Solid Edge part; units mm, degrees
sketch "Sketch1" plane through (0, 0, 0) normal (0, -1, 0) x (1, 0, 0)
  line L0 (-39.1421, 0) -> (39.1421, 0)
  line L1 (39.1421, 0) -> (91.1421, 52)
  line L2 (91.1421, 52) -> (77, 52)
  line L3 (77, 52) -> (30, 5)
  line L4 (30, 5) -> (-30, 5)
  line L5 (-30, 5) -> (-77, 52)
  line L6 (-77, 52) -> (-91.1421, 52)
  line L7 (-91.1421, 52) -> (-39.1421, 0)
  dimension "D1" = 30
extrude "Protrusion1" add sketch "Sketch1" along normal blind 94.9203
sketch "Sketch2" plane through (0, -94.9203, 21) normal (0, -1, 0) x (1, 0, 0)
  line L0 (-86.1421, 26) -> (-91.1421, 31)
  line L1 (-101.1421, 26) -> (-86.1421, 26)
  line L2 (-101.1421, 31) -> (-101.1421, 26)
  line L3 (-91.1421, 31) -> (-101.1421, 31)
  dimension "D1" = 91.1421
  dimension "D2" = 101.1421
extrude "Protrusion2" add sketch "Sketch2" against normal up to vertex (94.9203 mm away)
mirror "Mirror1" about plane through (0, 0, 0) normal (1, 0, 0) of "Protrusion2"
sketch "Sketch3" plane through (0, -47.4602, 5) normal (0, 0, 1) x (1, 0, 0)
  circle A0 centre (-16, 21) radius 2
  circle A1 centre (-16, -21) radius 2
  circle A2 centre (16, -21) radius 2
  circle A3 centre (16, 21) radius 2
  dimension "D1" = 16
  dimension "D2" = 16
extrude "Cutout1" cut sketch "Sketch3" against normal through all
sketch "Sketch4" plane through (-78.2221, -47.4602, 52) normal (0, 0, 1) x (1, 0, 0)
  circle A0 centre (-17.7801, -40) radius 1.5
  circle A1 centre (174.2242, -40) radius 1.5
  circle A2 centre (174.2242, 40) radius 1.5
  circle A3 centre (-17.7801, 40) radius 1.5
  dimension "D1" = 17.7801
extrude "Cutout2" cut sketch "Sketch4" against normal through all
properties material "Nylon, allgemein"
The model under review builds one solid part; all positions refer to its coordinate system, in mm. A direction names the side the tool comes from. Round coordinates to 2 decimals unless told otherwise and drop trailing zeros. Loops run counter-clockwise (first coordinate to the right, second up) from the corner with the lowest first, then second, coordinate; pieces in that order, holes last. Notation, with made-up numbers: (28, 59.5) -> (32, 59.5) arc R13 ccw to (32, 71.5) -> close; hole circle Ø9 at (-9.5, 10). An arc over 180 degrees is marked (long way). Answer as a JSON object with one key per item and string values. Group by question number.
1) For faces 1 (the face through (0, -47, 5)), 2 (the face through (-94, -48, 47)), 3 (the face through (-1, -47, 0)), 4 (the face through (94, -48, 47)), list the 3-axis set-ups (+Z, -Z, +X, -X, +Y, -Y) from which the entire face can be reached by the end or side of a thin tool; tool diameter is ignored.
2) We need section D-D on x = 34. Write out the cut boundary in (y, z), then the cut area to 3 significant figures.
3) For pin 1 Ø7.5 at (x, y) = (-93.5, -56.5) entering from -Z; pin 2 Ø5 at (y, z) = (-81.5, 33.5) entering from +X; pin 3 Ø4 at (y, z) = (-20.5, 28) entering from +X, all flat-tipped, find the tip position at first contact; note any pin that passes through.
4) We need section C-C on z = 43. Write out the cut boundary in (x, y), then the cut area to 3 significant figures.
5) Mouldability with a two-part tool opening along X and no side actions: class faces 5 (the face through (89, -47, 52)), 6 (the face through (101.142, -48, 49)), 7 (the face through (15.566, -70.413, 2.535)) as released by +X, released by -X, zero draft, split by the parting line, or undercut.
6) We need section B-B on y = -43.5. Write out the cut boundary in (x, z), then the cut area to 3 significant figures.
7) We need section A-A on x = -16. Write out the cut boundary in (y, z).
8) For line 1 (Y direction, x = -16, z = 3.6); line 2 (X direction, y = -63, z = 29); line 3 (Z direction, x = 93.5, y = -38), list the stretches that pass through material, from the lowest coordinate up. Write a range as [from, to].
Result set:
{
 "1": {"face 1": "+Z, +Y, -Y", "face 2": "-Z, -X, +Y, -Y", "face 3": "-Z, +X, -X, +Y, -Y", "face 4": "-Z, +X, +Y, -Y"},
 "2": {"outline": "(-94.92, 0) -> (0, 0) -> (0, 9) -> (-94.92, 9) -> close", "area": "854 mm²"},
 "3": {"pin 1": "z = 47", "pin 2": "x = 75.14", "pin 3": "x = 69.14"},
 "4": {"outline": "(-82.14, -94.92) -> (-68, -94.92) -> (-68, 0) -> (-82.14, 0) -> close; (68, -94.92) -> (82.14, -94.92) -> (82.14, 0) -> (68, 0) -> close", "area": "2,680 mm²"},
 "5": {"face 5": "zero draft", "face 6": "released by +X", "face 7": "undercut"},
 "6": {"outline": "(-101.14, 47) -> (-86.14, 47) -> (-39.14, 0) -> (39.14, 0) -> (86.14, 47) -> (101.14, 47) -> (101.14, 52) -> (77, 52) -> (30, 5) -> (-30, 5) -> (-77, 52) -> (-101.14, 52) -> close", "area": "1,870 mm²"},
 "7": {"outline": "(-94.92, 0) -> (-70.46, 0) -> (-70.46, 5) -> (-94.92, 5) -> close; (-66.46, 0) -> (-28.46, 0) -> (-28.46, 5) -> (-66.46, 5) -> close; (-24.46, 0) -> (0, 0) -> (0, 5) -> (-24.46, 5) -> close"},
 "8": {"line 1": "[-94.92, -70.46], [-66.46, -28.46], [-24.46, 0]", "line 2": "[-68.14, -54], [54, 68.14]", "line 3": "[47, 52]"}
}
